from build123d import *

# Parameters (mm, degrees)
SKETCH_1_R         = 13
EXTRUDE_1545_DEPTH = 16
EXTRUDE_1_DEPTH    = 16


with BuildPart() as part:
    # 草图1 → Extrude 1545 (new body)
    with BuildSketch(Plane.XY):
        Polygon((730, -330), (520, -760), (380, -760), (0, -680), (0, -482.786642105), (110, 0), (730, 0), align=None)
        with Locations((510, -70)):
            Circle(SKETCH_1_R, mode=Mode.SUBTRACT)
        with Locations((590, -70)):
            Circle(SKETCH_1_R, mode=Mode.SUBTRACT)
        with Locations((670, -70)):
            Circle(SKETCH_1_R, mode=Mode.SUBTRACT)
        with Locations((510, -150)):
            Circle(SKETCH_1_R, mode=Mode.SUBTRACT)
        with Locations((590, -150)):
            Circle(SKETCH_1_R, mode=Mode.SUBTRACT)
        with Locations((670, -150)):
            Circle(SKETCH_1_R, mode=Mode.SUBTRACT)
        with Locations((510, -230)):
            Circle(SKETCH_1_R, mode=Mode.SUBTRACT)
        with Locations((590, -230)):
            Circle(SKETCH_1_R, mode=Mode.SUBTRACT)
        with Locations((670, -230)):
            Circle(SKETCH_1_R, mode=Mode.SUBTRACT)
        with Locations(Location((230, -230, 0), (0, 0, 180))):
            Circle(SKETCH_1_R, mode=Mode.SUBTRACT)
        with Locations(Location((310, -230, 0), (0, 0, 180))):
            Circle(SKETCH_1_R, mode=Mode.SUBTRACT)
        with Locations(Location((390, -230, 0), (0, 0, 180))):
            Circle(SKETCH_1_R, mode=Mode.SUBTRACT)
        with Locations(Location((230, -150, 0), (0, 0, 180))):
            Circle(SKETCH_1_R, mode=Mode.SUBTRACT)
        with Locations(Location((310, -150, 0), (0, 0, 180))):
            Circle(SKETCH_1_R, mode=Mode.SUBTRACT)
        with Locations(Location((390, -150, 0), (0, 0, 180))):
            Circle(SKETCH_1_R, mode=Mode.SUBTRACT)
        with Locations(Location((230, -70, 0), (0, 0, 180))):
            Circle(SKETCH_1_R, mode=Mode.SUBTRACT)
        with Locations(Location((310, -70, 0), (0, 0, 180))):
            Circle(SKETCH_1_R, mode=Mode.SUBTRACT)
        with Locations(Location((390, -70, 0), (0, 0, 180))):
            Circle(SKETCH_1_R, mode=Mode.SUBTRACT)
        with Locations((150, -70)):
            Circle(SKETCH_1_R, mode=Mode.SUBTRACT)
        with Locations((150, -150)):
            Circle(SKETCH_1_R, mode=Mode.SUBTRACT)
        with Locations((150, -230)):
            Circle(SKETCH_1_R, mode=Mode.SUBTRACT)
        with Locations((590, -370)):
            Circle(SKETCH_1_R, mode=Mode.SUBTRACT)
        with Locations((510, -370)):
            Circle(SKETCH_1_R, mode=Mode.SUBTRACT)
        with Locations(Location((390, -370, 0), (0, 0, 180))):
            Circle(SKETCH_1_R, mode=Mode.SUBTRACT)
        with Locations(Location((310, -370, 0), (0, 0, 180))):
            Circle(SKETCH_1_R, mode=Mode.SUBTRACT)
        with Locations((506, -470)):
            Circle(SKETCH_1_R, mode=Mode.SUBTRACT)
        with Locations((506, -550)):
            Circle(SKETCH_1_R, mode=Mode.SUBTRACT)
        with Locations((506, -630)):
            Circle(SKETCH_1_R, mode=Mode.SUBTRACT)
        with Locations((506, -710)):
            Circle(SKETCH_1_R, mode=Mode.SUBTRACT)
        with Locations(Location((394, -710, 0), (0, 0, 180))):
            Circle(SKETCH_1_R, mode=Mode.SUBTRACT)
        with Locations(Location((394, -630, 0), (0, 0, 180))):
            Circle(SKETCH_1_R, mode=Mode.SUBTRACT)
        with Locations(Location((394, -550, 0), (0, 0, 180))):
            Circle(SKETCH_1_R, mode=Mode.SUBTRACT)
        with Locations(Location((394, -470, 0), (0, 0, 180))):
            Circle(SKETCH_1_R, mode=Mode.SUBTRACT)
        with Locations((149.479377198, -397.484050539)):
            Circle(SKETCH_1_R, mode=Mode.SUBTRACT)
        with Locations((99.493096694, -459.945012437)):
            Circle(SKETCH_1_R, mode=Mode.SUBTRACT)
        with Locations((49.506816189, -522.405974336)):
            Circle(SKETCH_1_R, mode=Mode.SUBTRACT)
        with Locations((61.981497584, -634.85321674)):
            Circle(SKETCH_1_R, mode=Mode.SUBTRACT)
        with Locations((111.967778088, -572.392254841)):
            Circle(SKETCH_1_R, mode=Mode.SUBTRACT)
        with Locations((161.954058593, -509.931292942)):
            Circle(SKETCH_1_R, mode=Mode.SUBTRACT)
        with Locations((211.940339097, -447.470331043)):
            Circle(SKETCH_1_R, mode=Mode.SUBTRACT)
        with Locations(Location((174.428739987, -622.378535345, 0), (0, 0, 180))):
            Circle(SKETCH_1_R, mode=Mode.SUBTRACT)
        with Locations(Location((224.415020492, -559.917573446, 0), (0, 0, 180))):
            Circle(SKETCH_1_R, mode=Mode.SUBTRACT)
        with Locations(Location((274.401300996, -497.456611548, 0), (0, 0, 180))):
            Circle(SKETCH_1_R, mode=Mode.SUBTRACT)
    extrude(amount=EXTRUDE_1545_DEPTH)

    # 草图2 → 凸台-拉伸1 (add)
    with BuildSketch(Plane.XY.offset(16)):
        Polygon((110, 0), (730, 0), (730, -330), (520, -760), (380, -760), (0, -680), (0, -482.786642105), align=None)
    extrude(amount=-EXTRUDE_1_DEPTH)


solid = part.part
Here's how the part is built. I have some questions about the finished solid (model axes, mm). Coordinates: 2 decimals unless noted, no trailing zeros. Loops run counter-clockwise (first coordinate to the right, second up) from the corner with the lowest first, then second, coordinate; pieces in that order, holes last.
1. Imagine slicing it at C-C, the plane x = 213. Please give me the cut outline in (y, z).
2. Imagine slicing it at B-B, the plane y = -311.5. Please give me the cut outline in (x, z).
3. I need wall thicknesses on L1, parallel to Y at x = 681, z = 5; L2, parallel to X at y = -654, z = 10.5; L3, parallel to Y at x = 626, z = 8.5. Which ranges of each line are inside material? Lowest first, please.
4. Imagine slicing it at A-A, the plane z = 5.75. Please give me the cut outline in (x, y).
5. For P1, Ø3, axis at y = -369.5, z = 13.5, coming from the -X side; P2, Ø2, axis at y = -458, z = 10, coming from the -X side; P3, Ø1.5, axis at y = -393, z = 10.5, coming from the +X side, each with a flat end and sliding along its axis, tell me the tip position at first contact or that it passes through.
6. If we mould it in two halves opening along Z, with no side actions, what happens to faces 1 (the flat face through (0, -583, 8)), 2 (the flat face through (370, -375, 0)), 3 (the flat face through (370, -375, 16))? For each: pulls with the +Z half, pulls with the -Z half, needs draft (parallel to the pull), parting line crosses it, or undercut.
Taken from the geometry:
1. outline: (-724.84, 0) - (0, 0) - (0, 16) - (-724.84, 16) - close
2. outline: (39.03, 0) - (730, 0) - (730, 16) - (39.03, 16) - close
3. L1: y = -430.33 to 0
3. L2: x = 0 to 571.77
3. L3: y = -542.95 to 0
4. outline: (0, -680) - (380, -760) - (520, -760) - (730, -330) - (730, 0) - (110, 0) - (0, -482.79) - close
5. P1: stops at x = 25.47
5. P2: stops at x = 5.42
5. P3: stops at x = 699.6
6. face 1: needs draft
6. face 2: pulls with the -Z half
6. face 3: pulls with the +Z half
